Autodesk Inventor part; units mm, degrees
ref_plane "Work Plane1" through (0, 27, 0) normal (0, 1, 0) x (-1, 0, 0)
ref_plane "YZ Plane" through (0, 0, 0) normal (1, 0, 0) x (0, 1, 0)
ref_plane "XY Plane" through (0, 0, 0) normal (0, 0, 1) x (1, 0, 0)
sketch "Sketch1" plane through (0, 0, 0) normal (0, 0, 1) x (1, 0, 0)
  line L0 (0, 0) -> (-27, 0)
  line L1 (-27, 0) -> (-27, 27)
  arc A0 (-24, 9) -> (-18, 3) centre (-18, 9) ccw
  arc A1 (-27, 9) -> (-18, 0) centre (-18, 9) ccw
  line L2 (0, 3) -> (-18, 3)
  line L3 (-24, 9) -> (-24, 27)
  line L4 (0, 0) -> (0, 3)
  line L5 (-27, 27) -> (-24, 27)
  line L6 (-25.5, 9) -> (-25.5, 27)
  line L7 (-18, 1.5) -> (0, 1.5)
  arc A2 (-25.5, 9) -> (-18, 1.5) centre (-18, 9) ccw
  line L8 (-24, 9) -> (-27, 9)
  line L9 (-18, 3) -> (-18, 0)
  dimension "d0" = 27
  dimension "d1" = 27
  dimension "d2" = 6
  dimension "d3" = 9
sketch "Sketch2" plane through (0, 0, 0) normal (1, 0, 0) x (0, 1, 0)
  circle A0 centre (1.5, 0) radius 1.5
  line L0 (0, 5.6966) -> (0, -5.6966) construction
  line L1 (3, 0) -> (-1.1636, 0) construction
  point P0 (0, 0)
  point P1 (0, 0)
  dimension "d5" = 3
  dimension "d6" = 1.5
ref_plane "Work Plane1" through (0, 27, 0) normal (0, 1, 0) x (-1, 0, 0)
sketch "Sketch3" plane through (0, 27, 0) normal (0, 1, 0) x (-1, 0, 0)
  circle A0 centre (25.5, 0) radius 1.5
  line L0 (27, 6.8213) -> (27, -6.8213) construction
  line L1 (30.5412, 0) -> (-1.145, 0) construction
  point P0 (0, 0)
  point P1 (27, 0)
  dimension "d8" = 3
  dimension "d9" = 27
  dimension "d10" = 25.5
sweep "Sweep1" add profiles "Sketch3" path "Sketch1" path curves L6 A2 L7
shell "Shell1" thickness 0.2 removed faces 2 at (0, 1.8952, 0.8627) at (-25.3633, 27, 0.3027)
properties part number "Hudson 1-70"
Check sheet for the modelled part. Datum: model origin and axes. Units: mm. Coordinates: 2 decimals unless noted, no trailing zeros. Write each loop counter-clockwise with the first axis right and the second up, starting at its lowest first coordinate (ties: lowest second). Pieces come first, ordered by that corner, then holes.
Item 1: Cross-section at A-A on z = 0. Record the boundary of the cut face in (x, y), then the cut area to 3 significant figures.
Numbers:
outline: (-27, 9) arc R9 ccw to (-18, 0) - (0, 0) - (0, 0.2) - (-18, 0.2) arc R8.8 cw to (-26.8, 9) - (-26.8, 27) - (-27, 27) - close; (-24.2, 9) arc R6.2 ccw to (-18, 2.8) - (0, 2.8) - (0, 3) - (-18, 3) arc R6 cw to (-24, 9) - (-24, 27) - (-24.2, 27) - close
area: 19.1 mm2
Item 2: Mould release check, pull along Y, two halves, no side actions. Record for faces 1 (the face through (-9.13, 2.8, 0.06)), 2 (the face through (-9.1, 2.7, -0.9)), 3 (the face through (-24, 18, 0)): released by +Y, released by -Y, zero draft, split by the parting line, or undercut.
Numbers:
face 1: undercut
face 2: split by the parting line
face 3: zero draft
Item 3: Scan lines: probe 1 along X at (y, z) = (21, 0); probe 2 along Y at (x, z) = (-9.25, -0.2); probe 3 along X at (y, z) = (4.75, -0.85). Record each from-to range of solid material in increasing order.
Numbers:
probe 1: x = -27 to -26.8, -24.2 to -24
probe 2: y = 0.01 to 0.22, 2.78 to 2.99
probe 3: x = -25.63 to -25.34, -22.94 to -22.6
Item 4: Cross-section at B-B on y = 14.75. Record the boundary of the cut face in (x, z).
Numbers:
outline: circle Ø3 at (-25.5, 0); hole circle Ø2.6 at (-25.5, 0)
Item 5: Depth check by flat-ended pin: pin 1 Ø1 at (y, z) = (19.5, -1) entering from +X. Enter the tip coordinate at first touch or a pass-through.
Numbers:
pin 1: stops at x = -24.09
Item 6: Cross-section at C-C on x = -15. Record the boundary of the cut face in (y, z), then the cut area to 3 significant figures.
Numbers:
outline: circle Ø3 at (1.5, 0); hole circle Ø2.6 at (1.5, 0)
area: 1.76 mm2
